from build123d import *

# Parameters (mm, degrees)
F0_W            = 76.2
F0_H            = 93.6498
F1_DEPTH        = 9.525
F2_W            = 40.259
F2_H            = 19.05
F3_DEPTH        = 15.875
F4_R            = 7.14375
F5_DEPTH        = 9.526
F6_R            = 6.35
F7_DEPTH        = 9.526
F8_R            = 6.35
F9_DEPTH        = 25.401
F10_R           = 2.38125
F11_DEPTH       = 9.526
F12_SIZE        = 6.35
F14_D           = 4.4958
F14_CBORE_D     = 7.9375
F14_CBORE_DEPTH = 4.1656
F16_D           = 3.4544
F16_CBORE_D     = 6.35
F16_CBORE_DEPTH = 3.175
F18_D           = 2.5908


with BuildPart() as f1:
    # F0 (on Front) → F1 (new body)
    with BuildSketch(Plane.XZ):
        Rectangle(F0_W, F0_H)
    extrude(amount=F1_DEPTH)

    # F2 (on face) → F3 (join)
    with BuildSketch(Plane.XZ.offset(9.525)):
        with Locations((0, 27.2923)):
            Rectangle(F2_W, F2_H)
    extrude(amount=F3_DEPTH)

    # F4 (on face) → F5 (cut, through all)
    with BuildSketch(Plane.XZ.offset(9.525)):
        with Locations((0, 5.5753)):
            Circle(F4_R)
    extrude(amount=-F5_DEPTH, mode=Mode.SUBTRACT)

    # F6 (on face) → F7 (cut, through all)
    with BuildSketch(Plane.XZ.offset(9.525)):
        with Locations((0, -10.2997)):
            Circle(F6_R)
    extrude(amount=-F7_DEPTH, mode=Mode.SUBTRACT)

    # F8 (on face) → F9 (cut, through all)
    with BuildSketch(Plane.XZ.offset(25.4)):
        with Locations((-12.7, 25.7175)):
            Circle(F8_R)
        with Locations((12.7, 25.7175)):
            Circle(F8_R)
    extrude(amount=-F9_DEPTH, mode=Mode.SUBTRACT)

    # F10 (on face) → F11 (cut, through all)
    with BuildSketch(Plane.XZ.offset(9.525)):
        with Locations((-27.94, -34.1249)):
            Circle(F10_R)
        with Locations((27.94, -34.1249)):
            Circle(F10_R)
    extrude(amount=-F11_DEPTH, mode=Mode.SUBTRACT)

    # F12
    f12_edges = [f1.edges().sort_by_distance(p)[0] for p in [
        (38.1, -4.7625, 46.8249),
        (-38.1, -4.7625, 46.8249),
    ]]
    chamfer(f12_edges, length=F12_SIZE)

    # F14 (through all)
    with Locations(Plane.XZ.offset(9.525)):
        with Locations((-31.75, -27.7749), (-31.75, -40.4749), (31.75, -40.4749), (31.75, -27.7749), (0, -27.7749), (0, -40.4749)):
            CounterBoreHole(F14_D / 2, F14_CBORE_D / 2, F14_CBORE_DEPTH)

    # F16 (through all)
    with Locations(Plane.XZ.offset(9.525)):
        with Locations((-25.4, 42.8625), (25.4, 42.8625), (34.1376, 13.5001), (34.1376, -11.8999), (-34.1376, -11.8999), (-34.1376, 13.5001)):
            CounterBoreHole(F16_D / 2, F16_CBORE_D / 2, F16_CBORE_DEPTH)

    # F18 (through all)
    with Locations(Plane.XZ.offset(9.525)):
        with Locations((-34.1376, 0.8001)):
            Hole(F18_D / 2)


solid = f1.part
Can you work these out from the model? Positions are in its coordinate system, mm. A direction names the side the tool comes from. Coordinates: 2 decimals unless noted, no trailing zeros. Loops run counter-clockwise (first coordinate to the right, second up) from the corner with the lowest first, then second, coordinate; pieces in that order, holes last. Notation, with made-up numbers: (41, -21.5) - (96, -21.5) arc R27 cw to (96, 10.5) - close; hole circle Ø11 at (-23, -20). An arc over 180 degrees is marked (long way). Put each result on its own line as item: value. Start each with the question number.
Item 1: Suppose I cut it at A-A (x = 12.7). Please give me the cut outline in (y, z) (1 decimal), and give its area (3 significant figures).
Item 2: If I drill on line 1 along Z through (x, y) = (31.75, -4.2); line 2 along Z through (x, y) = (25.4, -8.75); line 3 along Z through (x, y) = (31.75, -7.65), over which ranges is the centre line in solid material (lowest first)?
Item 3: Suppose I cut it at D-D (y = -17.5). Please give me the cut outline in (x, z), and give its area (3 significant figures).
Item 4: Suppose I cut it at B-B (x = 0). State how many separate pieces and enclosed holes the cut face has, and give its area (3 significant figures).
Item 5: Which directions (+Z, -Z, +X, -X, +Y, -Y) give clear straight access to the entire face, cutting with the end or side of a thin tool? Please do faces 5 (the face through (-1, -5, -46.825)), 6 (the face through (37.166, -7.96, 14.454)).
Item 6: For pin 1 (2 mm diameter, centred on x = 2.5, z = -24, fed in from -Y) (3 decimals); pin 2 (3 mm diameter, centred on x = 33, z = 14, fed in from -Y); pin 3 (1.5 mm diameter, centred on x = -10, z = 22, fed in from +Y); pin 4 (10 mm diameter, centred on x = -20, y = -17.5, fed in from +Z), each with a flat end and sliding along its axis, tell me the tip position at first contact or that it passes through.
Item 7: If we mould it in two halves opening along X, with no side actions, what happens to faces 1 (the face through (38.1, -5, -4)), 2 (the face through (-9, 0, 1)), 3 (the face through (-30.09, -2.64, -38.96)), 4 (the face through (-20.13, -17, 27))? For each: +X half, -X half, draft (parallel to the pull), parting line (faces both ways), or undercut.
Here are the results:
1. outline: (-25.4, 17.8) - (-9.5, 17.8) - (-9.5, -46.8) - (0, -46.8) - (0, 19.4) - (-25.4, 19.4) - close; (-25.4, 32.1) - (0, 32.1) - (0, 46.8) - (-9.5, 46.8) - (-9.5, 36.8) - (-25.4, 36.8) - close
1. area: 872 mm²
2. line 1: -46.82 to -42.72, -38.23 to -30.02, -25.53 to 46.82
2. line 2: -46.82 to 39.69, 46.04 to 46.82
2. line 3: -46.82 to -44.44, -36.51 to -31.74, -23.81 to -13.99, -9.81 to 11.41, 15.59 to 46.82
3. outline: (-20.13, 17.77) - (20.13, 17.77) - (20.13, 36.82) - (-20.13, 36.82) - close; hole circle Ø12.7 at (-12.7, 25.72); hole circle Ø12.7 at (12.7, 25.72)
3. area: 514 mm²
4. separate pieces: 5
4. enclosed holes: 0
4. area: 823 mm²
5. face 5: -Z, +X, -X, +Y, -Y
5. face 6: -Y
6. pin 1: y = -9.525
6. pin 2: y = -6.35
6. pin 3: through
6. pin 4: z = 36.82
7. face 1: +X half
7. face 2: draft
7. face 3: undercut
7. face 4: -X half
